from build123d import *

# Parameters (mm, degrees)
F2_SIZE = 0.8
F3_R    = 0.12


with BuildPart() as f1:
    # F0 (on Top) → F1 (revolve)
    with BuildSketch(Plane.XY):
        Polygon((-15.994198, 12.7), (-19.794198, 12.7), (-19.794198, 8.3), (-14.294198, 8.3), (-14.294198, 9.25), (-15.994198, 9.25), align=None)
    revolve(axis=Axis((-19.380304, 0, 0), (1, 0, 0)))

    # F2
    f2_edges = [f1.edges().sort_by_distance(p)[0] for p in [
        (-19.794198, -8.3, 0),
        (-19.794198, -12.7, 0),
    ]]
    chamfer(f2_edges, length=F2_SIZE)

    # F3
    f3_edges = [f1.edges().sort_by_distance(p)[0] for p in [
        (-15.994198, -9.25, 0),
        (-14.294198, -9.25, 0),
        (-15.994198, -12.7, 0),
    ]]
    fillet(f3_edges, radius=F3_R)


solid = f1.part
Can you work these out from the model? Positions are in its coordinate system, mm. Round coordinates to 2 decimals unless told otherwise and drop trailing zeros. Write each loop counter-clockwise with the first axis right and the second up, starting at its lowest first coordinate (ties: lowest second). Pieces come first, ordered by that corner, then holes. Notation, with made-up numbers: (88, 62.5) -> (96, 62.5) arc R18 cw to (96, 77.5) -> close; hole circle Ø2 at (67, 73.25). An arc over 180 degrees is marked (long way). One line per question, with ' | ' between items. Start each with the question number.
1) Suppose I cut it at A-A on z = 0. Write out the boundary of the cut face in (x, y), then the cut area to 3 significant figures.
2) I need wall thicknesses on line 1 (Z direction, x = -18, y = 0); line 2 (X direction, y = -4.75, z = 9.25); line 3 (Y direction, x = -16.4, z = -1.25). Which ranges of each line are inside material? Lowest first, please. Write a range as [from, to].
3) I'm going to push flat-ended pins straight in: P1, Ø3, axis at y = -6, z = 5, coming from the +X side; P2, Ø6, axis at y = 0, z = 2.5, coming from the -X side; P3, Ø1, axis at x = -17.5, y = 6, coming from the -Z side; P4, Ø3, axis at x = -19, y = -2, coming from the +Z side. Where does each tip first touch, or does it pass through?
4) Suppose I cut it at C-C on x = -16.55. Write out the boundary of the cut face in (y, z), then the cut area to 3 significant figures.
5) Suppose I cut it at D-D on x = -15.05. Write out the boundary of the cut face in (y, z).
6) If we mould it in two halves opening along Y, with no side actions, what happens to faces 1 (the cylindrical face through (-15.15, -2.01, -9.03)), 2 (the flat face through (-15.994, 1.9, 9.4)), 3 (the cylindrical face through (-16.611, -1.799, -8.103))? For each: released by +Y, released by -Y, zero draft, split by the parting line, or undercut.
Return value:
1) outline: (-19.79, -11.9) -> (-18.99, -12.7) -> (-16.11, -12.7) arc R0.12 ccw to (-15.99, -12.58) -> (-15.99, -9.37) arc R0.12 cw to (-15.87, -9.25) -> (-14.41, -9.25) arc R0.12 ccw to (-14.29, -9.13) -> (-14.29, -8.3) -> (-18.99, -8.3) -> (-19.79, -9.1) -> close; (-19.79, 9.1) -> (-18.99, 8.3) -> (-14.29, 8.3) -> (-14.29, 9.13) arc R0.12 ccw to (-14.41, 9.25) -> (-15.87, 9.25) arc R0.12 cw to (-15.99, 9.37) -> (-15.99, 12.58) arc R0.12 ccw to (-16.11, 12.7) -> (-18.99, 12.7) -> (-19.79, 11.9) -> close | area: 35.4 mm2
2) line 1: z = [-12.7, -8.3], [8.3, 12.7] | line 2: x = [-19.79, -15.99] | line 3: y = [-12.64, -8.21], [8.21, 12.64]
3) P1: stops at x = -14.29 | P2: passes through | P3: stops at z = -11.45 | P4: stops at z = 12.69
4) outline: circle Ø25.4 at (0, 0); hole circle Ø16.6 at (0, 0) | area: 290 mm2
5) outline: circle Ø18.5 at (0, 0); hole circle Ø16.6 at (0, 0)
6) face 1: split by the parting line | face 2: zero draft | face 3: undercut
